```python
from build123d import *

# Parameters (mm, degrees)
BOSS_EXTRUDE1_DEPTH = 7.62
SKETCH3_R           = 2.099999991
SKETCH3_R_2         = 2.1
CUT_EXTRUDE1_DEPTH  = 170.067196777
SKETCH3_3_R         = 2.1
CUT_EXTRUDE2_DEPTH  = 6.35
FILLET1_R           = 2


with BuildPart() as part:
    # Sketch2 → Boss-Extrude1 (new body)
    with BuildSketch(Plane(origin=(0, 0, -0.41148), x_dir=(-1, 0, 0), z_dir=(0, 0, -1))):
        Polygon((-92.964, 58.674), (-92.964, 50.673), (-138.811, 50.673), (-138.811, 58.674), (-147.701, 58.674), (-147.701, 66.294), (-147.701, 73.914), (-138.811, 73.914), (-138.811, 81.915), (-92.964, 81.915), (-92.964, 73.914), (-84.074, 73.914), (-84.074, 66.294), (-84.074, 58.674), align=None)
    extrude(amount=BOSS_EXTRUDE1_DEPTH)

    # Sketch3 → Cut-Extrude1 (cut, through all)
    with BuildSketch(Plane.XY.offset(-0.41148)):
        with Locations((88.524, 66.294)):
            Circle(SKETCH3_R)
        with Locations((143.251, 66.294)):
            Circle(SKETCH3_R_2)
    extrude(amount=-CUT_EXTRUDE1_DEPTH, mode=Mode.SUBTRACT)

    # Sketch3<3> → Cut-Extrude2 (cut)
    with BuildSketch(Plane.XY.offset(-0.41148)):
        with Locations((96.647, 78.232)):
            Circle(SKETCH3_3_R)
        with Locations((96.647, 54.356)):
            Circle(SKETCH3_3_R)
        with Locations((135.128, 54.356)):
            Circle(SKETCH3_3_R)
        with Locations((135.128, 78.232)):
            Circle(SKETCH3_3_R)
    extrude(amount=-CUT_EXTRUDE2_DEPTH, mode=Mode.SUBTRACT)

    # Fillet1
    fillet1_edges = [part.edges().sort_by_distance(p)[0] for p in [
        (138.811, 81.915, -4.22148),
        (92.964, 81.915, -4.22148),
        (84.074, 73.914, -4.22148),
        (84.074, 58.674, -4.22148),
        (92.964, 50.673, -4.22148),
        (138.811, 50.673, -4.22148),
        (147.701, 58.674, -4.22148),
        (147.701, 73.914, -4.22148),
    ]]
    fillet(fillet1_edges, radius=FILLET1_R)


solid = part.part
```
The model under review builds one solid part; all positions refer to its coordinate system, in mm. A direction names the side the tool comes from. Round coordinates to 2 decimals unless told otherwise and drop trailing zeros. Write each loop counter-clockwise with the first axis right and the second up, starting at its lowest first coordinate (ties: lowest second). Pieces come first, ordered by that corner, then holes. Notation, with made-up numbers: (48, -38.5) - (65, -38.5) arc R8 ccw to (65, -28.5) - close; hole circle Ø8 at (32, 15). An arc over 180 degrees is marked (long way). Use one line per item in the form item = value.
Q1. Tool access review of faces 4 (the flat face through (135, 54, -6.761)), 5 (the flat face through (90, 73.914, -4)), 6 (the flat face through (142, 73.914, -4)): name each direction out of +Z, -Z, +X, -X, +Y, -Y from which nothing blocks a thin tool from reaching the whole face with its end or side.
Answer key:
face_4 = +Z
face_5 = +Z, -Z, -X, +Y
face_6 = +Z, -Z, +X, +Y
Q2. Draft analysis for pull direction Y (two halves, no side actions). For faces 1 (the cylindrical face through (86.858, 65.016, -4.168)), 2 (the flat face through (147.701, 66, -4)), 3 (the cylindrical face through (147.1, 59.244, -4.275)), state which applies: +Y half, -Y half, draft (parallel to the pull), parting line (faces both ways), or undercut.
Answer key:
face_1 = undercut
face_2 = draft
face_3 = -Y half
Q3. Consider section A-A (z = -5.25). State the section outline as (x, y) points (3 decimals).
Answer key:
outline = (84.074, 60.674) arc R2 ccw to (86.074, 58.674) - (92.964, 58.674) - (92.964, 52.673) arc R2 ccw to (94.964, 50.673) - (136.811, 50.673) arc R2 ccw to (138.811, 52.673) - (138.811, 58.674) - (145.701, 58.674) arc R2 ccw to (147.701, 60.674) - (147.701, 71.914) arc R2 ccw to (145.701, 73.914) - (138.811, 73.914) - (138.811, 79.915) arc R2 ccw to (136.811, 81.915) - (94.964, 81.915) arc R2 ccw to (92.964, 79.915) - (92.964, 73.914) - (86.074, 73.914) arc R2 ccw to (84.074, 71.914) - close; hole circle Ø4.2 at (88.524, 66.294); hole circle Ø4.2 at (96.647, 54.356); hole circle Ø4.2 at (96.647, 78.232); hole circle Ø4.2 at (135.128, 54.356); hole circle Ø4.2 at (135.128, 78.232); hole circle Ø4.2 at (143.251, 66.294)
Q4. Consider section B-B (x = 89.5). State the section outline as (y, z) points, and give its area (3 significant figures).
Answer key:
outline = (58.67, -8.03) - (64.43, -8.03) - (64.43, -0.41) - (58.67, -0.41) - close; (68.15, -8.03) - (73.91, -8.03) - (73.91, -0.41) - (68.15, -0.41) - close
area = 87.8 mm2
Q5. For line 1 (X direction, y = 57, z = -5.5); line 2 (Y direction, x = 97, z = -5.5) (3 decimals); line 3 (Z direction, x = 95.5, y = 53.5), list the stretches that pass through material, from the lowest coordinate up. Write a range as [from, to].
Answer key:
line_1 = [92.96, 138.81]
line_2 = [50.673, 52.286], [56.426, 76.162], [80.302, 81.915]
line_3 = [-8.03, -6.76]
Q6. Consider section C-C (y = 58). State the section outline as (x, z) points, and give its area (3 significant figures).
Answer key:
outline = (92.96, -8.03) - (138.81, -8.03) - (138.81, -0.41) - (92.96, -0.41) - close
area = 349 mm2
Q7. Insertion check: pin 1 Ø1.8 at (y, z) = (77.5, -4) entering from -X; pin 2 Ø4 at (x, z) = (141, -2.5) entering from -Y; pin 3 Ø4 at (x, y) = (88.524, 66.294) entering from +Z; pin 4 Ø3.5 at (x, y) = (135.128, 78.232) entering from +Z. Each pin has a flat end and moves straight along its axis. Give the tip position at first contact, or say it passes through.
Answer key:
pin_1 = 92.96
pin_2 = 58.67
pin_3 = through
pin_4 = -6.76
